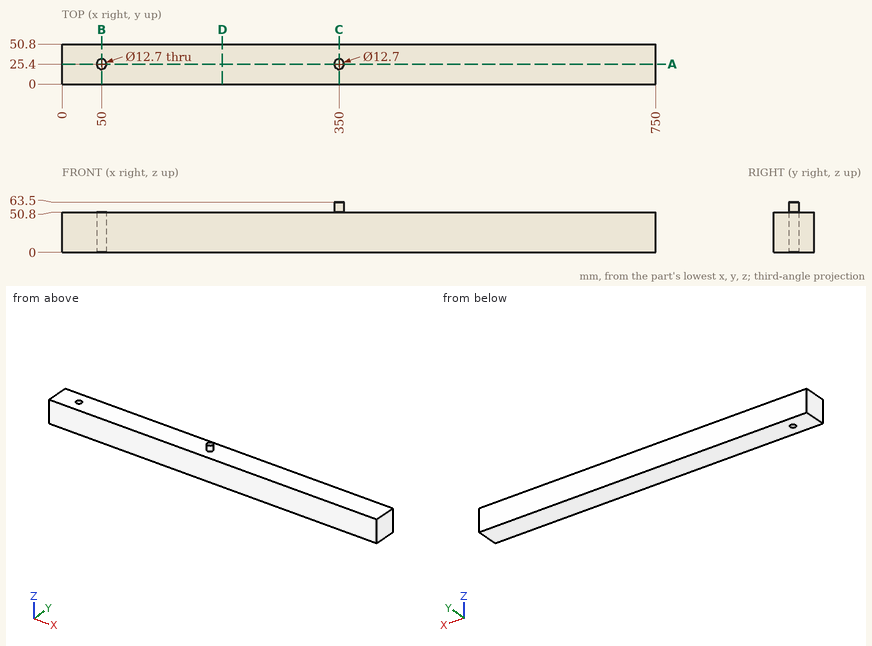
Geometry check sheet. Reference: drawing and pictorial views, mm from the part's lowest x, y, z. Coordinates: 2 decimals unless noted, no trailing zeros. Write each loop counter-clockwise with the first axis right and the second up, starting at its lowest first coordinate (ties: lowest second). Pieces come first, ordered by that corner, then holes. Notation, with made-up numbers: M 15.25,0 L 51.25,0 A23 cw 51.25,13 Z; hole C 25,63 d1. An arc over 180 degrees is marked long. Use one line per item in the form item = value.
Item 1: Sectioned sample at D-D, the plane x = 202.5. Record the cut outline in (y, z), and give its area (3 significant figures).
Answer below:
outline = M 0,0 L 50.8,0 L 50.8,50.8 L 0,50.8 Z
area = 2,580 mm^2
Item 2: Gauge pin test, flat end, axial feed: pin 1 Ø5 at (y, z) = (14.5, 45) entering from -X. Record the tip position at first contact, or that the pin passes through.
Answer below:
pin_1 = 0
Item 3: Sectioned sample at C-C, the plane x = 350. Record the cut outline in (y, z).
Answer below:
outline = M 0,0 L 50.8,0 L 50.8,50.8 L 31.75,50.8 L 31.75,63.5 L 19.05,63.5 L 19.05,50.8 L 0,50.8 Z
Item 4: Material ranges on L1, parallel to Y at x = 50, z = 25; L2, parallel to X at y = 24.5, z = 30.5; L3, parallel to Z at x = 305.5, y = 37, recorded low to high. Write a range as from..to.
Answer below:
L1 = 0..19.05, 31.75..50.8
L2 = 0..43.71, 56.29..750
L3 = 0..50.8
Item 5: Sectioned sample at A-A, the plane y = 25.4. Record the cut outline in (x, z).
Answer below:
outline = M 0,0 L 43.65,0 L 43.65,50.8 L 0,50.8 Z; M 56.35,0 L 750,0 L 750,50.8 L 356.35,50.8 L 356.35,63.5 L 343.65,63.5 L 343.65,50.8 L 56.35,50.8 Z
Item 6: Sectioned sample at B-B, the plane x = 50. Record the cut outline in (y, z), and give its area (3 significant figures).
Answer below:
outline = M 0,0 L 19.05,0 L 19.05,50.8 L 0,50.8 Z; M 31.75,0 L 50.8,0 L 50.8,50.8 L 31.75,50.8 Z
area = 1,940 mm^2
